from build123d import *

# Parameters (mm, degrees)
CROQUIS1_W                 = 101.6
CROQUIS1_H                 = 88.9
SALIENTE_EXTRUIR1_DEPTH    = 3
CORTAR_EXTRUIR1_DEPTH      = 136.036180337
CORTAR_EXTRUIR1_DEPTH_BACK = 136.036180337


with BuildPart() as part:
    # Croquis1 → Saliente-Extruir1 (new body)
    with BuildSketch(Plane(origin=(0, 0, 0), x_dir=(1, 0, 0), z_dir=(0, 1, 0))):
        with Locations((50.8, 44.45)):
            Rectangle(CROQUIS1_W, CROQUIS1_H)
    extrude(amount=SALIENTE_EXTRUIR1_DEPTH)

    # Croquis2 → Cortar-Extruir1 (cut, two sides: drawn at the far end of the back side and taken through both)
    with BuildSketch(Plane(origin=(101.6, 0, 0), x_dir=(0, 0, -1), z_dir=(1, 0, 0)).offset(-CORTAR_EXTRUIR1_DEPTH_BACK)):
        Polygon((88.9, 3), (88.9, 1.5), (78.9, 3), (78.9, 5.806097786), (88.9, 5.806097786), align=None)
    extrude(amount=CORTAR_EXTRUIR1_DEPTH + CORTAR_EXTRUIR1_DEPTH_BACK, mode=Mode.SUBTRACT)


solid = part.part
The listing builds one solid part. Answer for the finished solid, in the listing's coordinates (mm). Give positions to 0.01 mm unless a question says otherwise; leave off trailing zeros. Write each loop counter-clockwise with the first axis right and the second up, starting at its lowest first coordinate (ties: lowest second). Pieces come first, ordered by that corner, then holes.
1) Section A-A (x = 29.5) is taken. Write down the section's boundary in (y, z), and give its area (3 significant figures).
2) Section B-B (y = 2.3) is taken. Write down the section's boundary in (x, z), and give its area (3 significant figures).
3) Find the intervals of material crossed by L1, parallel to Y at x = 63, z = -83 (3 decimals), in increasing order.
Response:
1. outline: (0, -88.9) - (1.5, -88.9) - (3, -78.9) - (3, 0) - (0, 0) - close
1. area: 259 mm2
2. outline: (0, -83.57) - (101.6, -83.57) - (101.6, 0) - (0, 0) - close
2. area: 8,490 mm2
3. L1: y = 0 to 2.385
